The listing builds one solid part. Answer for the finished solid, in the listing's coordinates (mm). Face numbers are marked on the shaded views. Give positions to 0.01 mm unless a question says otherwise; leave off trailing zeros. Order: outer loops, then holes, each group sorted by start corner. A loop starts at its lowest first (then second) coordinate and runs counter-clockwise, first axis right, second up. Notation, with made-up numbers: (-10, 85) -> (39, 85) arc R24 cw to (39, 122) -> close; hole circle Ø6 at (-12.5, 63.5). An arc over 180 degrees is marked (long way). One line per question, with ' | ' between items. Start each with the question number.
```python
from build123d import *

# Parameters (mm, degrees)
SKETCH1_R           = 15
BOSS_EXTRUDE1_DEPTH = 105
SKETCH6_R           = 14.222015383
CUT_EXTRUDE4_DEPTH  = 3
SHELL1_START        = 3
SHELL1_OUTLINE_R    = 13.5
SHELL1_DEPTH        = 102
SKETCH8_R           = 14.157324042
CUT_EXTRUDE6_DEPTH  = 3
CUT_EXTRUDE7_START  = -20
CUT_EXTRUDE7_DEPTH  = 20


# Read off the part's stored shape, not the designer's step: Shell1
with BuildPart() as part:
    # Sketch1 → Boss-Extrude1 (new body)
    with BuildSketch(Plane(origin=(0, 0, 0), x_dir=(1, 0, 0), z_dir=(0, 1, 0))):
        with Locations(Location((0, 0, 0), (0, 0, 270))):
            Circle(SKETCH1_R)
    extrude(amount=BOSS_EXTRUDE1_DEPTH)

    # Sketch6 → Cut-Extrude4 (cut)
    with BuildSketch(Plane.XZ):
        with Locations(Location((0, 0, 0), (0, 0, 270))):
            Circle(SKETCH6_R)
    extrude(amount=-CUT_EXTRUDE4_DEPTH, mode=Mode.SUBTRACT)

    # Shell1 outline → Shell1 (cut)
    with BuildSketch(Plane(origin=(0, 0, 0), x_dir=(1, 0, 0), z_dir=(0, 1, 0)).offset(SHELL1_START)):
        Circle(SHELL1_OUTLINE_R)
    extrude(amount=SHELL1_DEPTH, mode=Mode.SUBTRACT)

    # Sketch8 → Cut-Extrude6 (cut)
    with BuildSketch(Plane(origin=(0, 105, 0), x_dir=(1, 0, 0), z_dir=(0, 1, 0))):
        with Locations(Location((0, 0, 0), (0, 0, 270))):
            Circle(SKETCH8_R)
    extrude(amount=-CUT_EXTRUDE6_DEPTH, mode=Mode.SUBTRACT)

    # Sketch9 → Cut-Extrude7 (cut)
    with BuildSketch(Plane(origin=(0, 105, 0), x_dir=(1, 0, 0), z_dir=(0, 1, 0)).offset(CUT_EXTRUDE7_START)):
        with BuildLine():
            Line((14.918575787, 1.560799953), (13.426718208, 1.404719958))
            Line((13.426718208, 1.404719958), (-13.47075587, 0.888108258))
            Line((-13.47075587, 0.888108258), (-14.925527409, 1.492860192))
            ThreePointArc((-14.925527409, 1.492860192), (-0.03414724, 14.999961132), (14.918575787, 1.560799953))
        make_face()
    extrude(amount=CUT_EXTRUDE7_DEPTH, mode=Mode.SUBTRACT)


solid = part.part
```
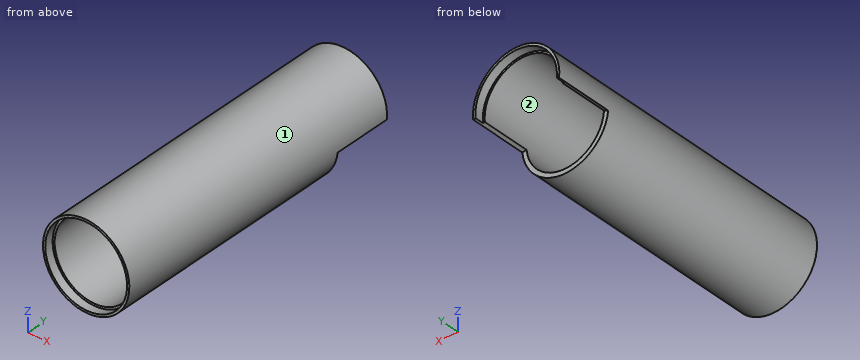
(1) Given P1, Ø5, axis at x = -2, z = -11, coming from the +Y side; P2, Ø3, axis at y = 30.5, z = 5.5, coming from the -X side; P3, Ø1, axis at x = 6, y = 53, coming from the -Z side, each flat-ended and moving along its own axis, determine where each tip first touches the part or whether it passes through.
(2) The part is cut by section C-C on z = -8.5. Determine the outline of the cut face in (x, y).
(3) The part is cut by section D-D on y = 88. Determine the outline of the cut face in (x, z).
(4) The part is cut by section A-A on x = 0. Determine the outline of the cut face in (y, z), plus the area to 3 significant figures.
(5) Consider line 1 (X direction, y = 67.5, z = 0); line 2 (X direction, y = 102.95, z = 0). Determine where each line is inside the solid, lowest interval first.
(6) Determine the mould class of the marked faces 1 and 2 for opening direction X: pulls with the +X half, pulls with the -X half, needs draft (parallel to the pull), parting line crosses it, or undercut.
(7) The part is cut by section B-B on y = 56. Determine the outline of the cut face in (x, z).
Result sheet:
1) P1: stops at y = 85 | P2: stops at x = -14.46 | P3: stops at z = -13.96
2) outline: (-12.36, 0) -> (-11.4, 0) -> (-11.4, 3) -> (-10.49, 3) -> (-10.49, 85) -> (-12.36, 85) -> close; (10.49, 3) -> (11.4, 3) -> (11.4, 0) -> (12.36, 0) -> (12.36, 85) -> (10.49, 85) -> close
3) outline: (-14.93, -1.49) -> (-13.47, -0.89) arc R13.5 cw (long way) to (13.43, -1.4) -> (14.92, -1.56) arc R15 ccw (long way) to start
4) outline: (0, -15) -> (85, -15) -> (85, -13.5) -> (3, -13.5) -> (3, -14.22) -> (0, -14.22) -> close; (0, 14.22) -> (3, 14.22) -> (3, 13.5) -> (102, 13.5) -> (102, 14.16) -> (105, 14.16) -> (105, 15) -> (0, 15) -> close | area: 279 mm^2
5) line 1: x = -15 to -13.5, 13.5 to 15 | line 2: x = -15 to -14.16, 14.16 to 15
6) face 1: parting line crosses it | face 2: undercut
7) outline: circle Ø30 at (0, 0); hole circle Ø27 at (0, 0)
